Read the model definition and answer for the solid it produces. Units are mm, in the model's axes. A direction names the side the tool comes from. Coordinates: 2 decimals unless noted, no trailing zeros. Loops run counter-clockwise (first coordinate to the right, second up) from the corner with the lowest first, then second, coordinate; pieces in that order, holes last. Notation, with made-up numbers: (0, 4) -> (44, 4) arc R33 ccw to (44, 38) -> close; hole circle Ø4 at (27.25, -17.75). An arc over 180 degrees is marked (long way). Answer in a Markdown table with one row per item.
```python
from build123d import *

# Parameters (mm, degrees)
SKETCH28_W                                   = 80
SKETCH28_H                                   = 80
BOSS_EXTRUDE1_DEPTH                          = 10
CBORE_FOR_M10_CHEESE_HEAD_SCREW1_D           = 12
CBORE_FOR_M10_CHEESE_HEAD_SCREW1_CBORE_D     = 26
CBORE_FOR_M10_CHEESE_HEAD_SCREW1_CBORE_DEPTH = 5
SKETCH36_R                                   = 1
BOSS_EXTRUDE5_DEPTH                          = 10
SKETCH37_R                                   = 22.5
SKETCH37_R_2                                 = 15.5
CUT_EXTRUDE2_DEPTH                           = 6
CUT_EXTRUDE6_DEPTH                           = 6
SKETCH40_W                                   = 18.062589032
SKETCH40_H                                   = 3
BOSS_EXTRUDE7_DEPTH                          = 13
SKETCH41_R                                   = 33.75
SKETCH41_R_2                                 = 26.25
CUT_EXTRUDE7_DEPTH                           = 1.65
SKETCH42_W                                   = 9.8
SKETCH42_H                                   = 11.037342061
CUT_EXTRUDE8_DEPTH                           = 2
CUT_EXTRUDE11_DEPTH                          = 20
SKETCH45_W                                   = 2.851047628
SKETCH45_H                                   = 9.955339391
BOSS_EXTRUDE8_DEPTH                          = 14
BOSS_EXTRUDE9_START                          = -9.955339
BOSS_EXTRUDE9_DEPTH                          = 9.955339


with BuildPart() as part:
    # Sketch28 → Boss-Extrude1 (new body)
    with BuildSketch(Plane(origin=(0, 0, 0), x_dir=(1, 0, 0), z_dir=(0, 1, 0))):
        with Locations((1.944585414, 4.241283073)):
            Rectangle(SKETCH28_W, SKETCH28_H)
    extrude(amount=BOSS_EXTRUDE1_DEPTH)

    # CBORE for M10 Cheese Head Screw1 (through all)
    with Locations(Plane(origin=(0, 10, 0), x_dir=(1, 0, 0), z_dir=(0, 1, 0))):
        with Locations((1.944585414, 4.241283073)):
            CounterBoreHole(CBORE_FOR_M10_CHEESE_HEAD_SCREW1_D / 2, CBORE_FOR_M10_CHEESE_HEAD_SCREW1_CBORE_D / 2, CBORE_FOR_M10_CHEESE_HEAD_SCREW1_CBORE_DEPTH)

    # Sketch36 → Boss-Extrude5 (add)
    with BuildSketch(Plane.XZ):
        with Locations(Location((12.444585414, -16.741283073, 0), (0, 0, 270))):
            Circle(SKETCH36_R)
        with Locations(Location((12.444585414, -4.241283073, 0), (0, 0, 270))):
            Circle(SKETCH36_R)
        with Locations(Location((-8.555414586, -16.741283073, 0), (0, 0, 90))):
            Circle(SKETCH36_R)
        with Locations(Location((-8.555414586, -4.241283073, 0), (0, 0, 90))):
            Circle(SKETCH36_R)
    extrude(amount=BOSS_EXTRUDE5_DEPTH)

    # Sketch37 → Cut-Extrude2 (cut)
    with BuildSketch(Plane(origin=(0, 10, 0), x_dir=(1, 0, 0), z_dir=(0, 1, 0))):
        with Locations(Location((1.944585414, 4.241283073, 0), (0, 0, 270))):
            Circle(SKETCH37_R)
        with Locations(Location((1.944585414, 4.241283073, 0), (0, 0, 270))):
            Circle(SKETCH37_R_2, mode=Mode.SUBTRACT)
    extrude(amount=-CUT_EXTRUDE2_DEPTH, mode=Mode.SUBTRACT)

    # Sketch39 → Cut-Extrude6 (cut)
    with BuildSketch(Plane(origin=(0, 10, 0), x_dir=(1, 0, 0), z_dir=(0, 1, 0))):
        with BuildLine():
            Line((6.944585414, -35.758716927), (6.944585414, -17.696127895))
            ThreePointArc((6.944585414, -17.696127895), (1.944585414, -18.258716927), (-3.055414586, -17.696127895))
            Line((-3.055414586, -17.696127895), (-3.055414586, -35.758716927))
            Line((-3.055414586, -35.758716927), (1.944585414, -35.758716927))
            Line((1.944585414, -35.758716927), (6.944585414, -35.758716927))
        make_face()
    extrude(amount=-CUT_EXTRUDE6_DEPTH, mode=Mode.SUBTRACT)

    # Sketch40 → Boss-Extrude7 (add)
    with BuildSketch(Plane(origin=(-3.055414586, 0, 0), x_dir=(0, 0, -1), z_dir=(1, 0, 0))):
        with Locations((-26.727422411, 8.5)):
            Rectangle(SKETCH40_W, SKETCH40_H)
    extrude(amount=BOSS_EXTRUDE7_DEPTH)

    # Sketch41 → Cut-Extrude7 (cut)
    with BuildSketch(Plane(origin=(0, 10, 0), x_dir=(1, 0, 0), z_dir=(0, 1, 0))):
        with Locations(Location((1.944585414, 4.241283073, 0), (0, 0, 270))):
            Circle(SKETCH41_R)
        with Locations(Location((1.944585414, 4.241283073, 0), (0, 0, 270))):
            Circle(SKETCH41_R_2, mode=Mode.SUBTRACT)
    extrude(amount=-CUT_EXTRUDE7_DEPTH, mode=Mode.SUBTRACT)

    # Sketch42 → Cut-Extrude8 (cut)
    with BuildSketch(Plane.XZ):
        with Locations((1.966640169, -13.109663986)):
            Rectangle(SKETCH42_W, SKETCH42_H)
    extrude(amount=-CUT_EXTRUDE8_DEPTH, mode=Mode.SUBTRACT)

    # Sketch43 → Cut-Extrude11 (cut)
    with BuildSketch(Plane(origin=(0, 10, 0), x_dir=(1, 0, 0), z_dir=(0, 1, 0))):
        with BuildLine():
            ThreePointArc((-38.055414586, 4.241282966), (-26.339685871, 32.525554283), (1.944585414, 44.241283073))
            Line((1.944585414, 44.241283073), (-38.055414586, 44.241283073))
            Line((-38.055414586, 44.241283073), (-38.055414586, 4.241282966))
        make_face()
        with BuildLine():
            ThreePointArc((1.944585414, -35.758716927), (-26.339685795, -24.042988212), (-38.055414586, 4.241282966))
            Line((-38.055414586, 4.241282966), (-38.055414586, -35.758716927))
            Line((-38.055414586, -35.758716927), (1.944585414, -35.758716927))
        make_face()
        with BuildLine():
            Line((41.944585414, -35.758716927), (41.944585414, 4.241283073))
            ThreePointArc((41.944585414, 4.241283073), (30.228856662, -24.042988174), (1.944585414, -35.758716927))
            Line((1.944585414, -35.758716927), (41.944585414, -35.758716927))
        make_face()
        with BuildLine():
            Line((41.944585414, 44.241283073), (1.944585414, 44.241283073))
            ThreePointArc((1.944585414, 44.241283073), (30.228856662, 32.525554321), (41.944585414, 4.241283073))
            Line((41.944585414, 4.241283073), (41.944585414, 44.241283073))
        make_face()
    extrude(amount=-CUT_EXTRUDE11_DEPTH, mode=Mode.SUBTRACT)

    # Sketch45 → Boss-Extrude8 (add)
    with BuildSketch(Plane(origin=(0, 8.35, 0), x_dir=(1, 0, 0), z_dir=(0, 1, 0))):
        with Locations((-32.810971356, 5.43037333)):
            Rectangle(SKETCH45_W, SKETCH45_H)
    extrude(amount=BOSS_EXTRUDE8_DEPTH)

    # Sketch46 → Boss-Extrude9 (add)
    with BuildSketch(Plane.XY.offset(-0.452703634).offset(BOSS_EXTRUDE9_START)):
        Polygon((-31.385447542, 22.35), (-31.385447542, 20.057188555), (-29.944471524, 20.057188555), align=None)
    extrude(amount=BOSS_EXTRUDE9_DEPTH)


solid = part.part
```
1. A cutting plane is placed at C-C on y = -5. Give the vertices of the cut face in (x, z), and give its area (3 significant figures).
A:
| item | result |
|---|---|
| outline | circle Ø2 at (-8.56, -16.74); circle Ø2 at (-8.56, -4.24); circle Ø2 at (12.44, -16.74); circle Ø2 at (12.44, -4.24) |
| area | 12.6 mm2 |
2. A cutting plane is placed at B-B on z = 10. Give the vertices of the cut face in (x, y), and give its area (3 significant figures).
A:
| item | result |
|---|---|
| outline | (-35.43, 0) -> (39.32, 0) -> (39.32, 10) -> (32.54, 10) -> (32.54, 8.35) -> (24, 8.35) -> (24, 10) -> (19.36, 10) -> (19.36, 4) -> (8.06, 4) -> (8.06, 10) -> (-4.17, 10) -> (-4.17, 4) -> (-15.47, 4) -> (-15.47, 10) -> (-20.11, 10) -> (-20.11, 8.35) -> (-28.65, 8.35) -> (-28.65, 10) -> (-35.43, 10) -> close |
| area | 584 mm2 |
3. A cutting plane is placed at D-D on y = 15. Give the vertices of the cut face in (x, z).
A:
| item | result |
|---|---|
| outline | (-34.24, -10.41) -> (-31.39, -10.41) -> (-31.39, -0.45) -> (-34.24, -0.45) -> close |
4. The mould has two halves that part along Y. Classify faces 1 (the cylindrical face through (9.829, 9.187, 20.797)), 2 (the flat face through (2, 7, 27)), 3 (the flat face through (15, 10, -1)): pulls with the +Y half, pulls with the -Y half, needs draft (parallel to the pull), parting line crosses it, or undercut.
A:
| item | result |
|---|---|
| face 1 | needs draft |
| face 2 | undercut |
| face 3 | pulls with the +Y half |
5. Given pin 1 Ø12 at (y, z) = (3, -31) entering from +X; pin 2 Ø1.3 at (x, y) = (-33, 14) entering from +Z; pin 3 Ø13 at (x, z) = (2, -5.5) entering from +Y, each flat-ended and moving along its own axis, determine where each tip first touches the part or whether it passes through.
A:
| item | result |
|---|---|
| pin 1 | stops at x = 36.14 |
| pin 2 | stops at z = -0.45 |
| pin 3 | stops at y = 5 |
6. A cutting plane is placed at A-A on x = -29. Give the vertices of the cut face in (y, z), and give its area (3 significant figures).
A:
| item | result |
|---|---|
| outline | (0, -29.59) -> (10, -29.59) -> (10, -17.71) -> (8.35, -17.71) -> (8.35, 9.23) -> (10, 9.23) -> (10, 21.1) -> (0, 21.1) -> close |
| area | 462 mm2 |
7. A tool of negligible diameter and unlimited length cuts with its end or side. For faces 4 (the flat face through (-2.933, 1, -13)), 5 (the cylindrical face through (-0.87, 7.54, 8.45)), 6 (the flat face through (7, 4, 11)), from which of +Z, -Z, +X, -X, +Y, -Y can it reach the whole face along a straight path? Write none if from no direction.
A:
| item | result |
|---|---|
| face 4 | -Y |
| face 5 | +Y |
| face 6 | none |
8. Find the intervals of material crossed by probe 1 along Z at (x, y) = (-0.5, 8.5); probe 2 along Y at (x, z) = (31.5, -0.5); probe 3 along Y at (x, z) = (-8, -7), in increasing order.
A:
| item | result |
|---|---|
| probe 1 | z = -44.17 to -37.9, -30.38 to -26.61, -19.55 to -17.01, 8.53 to 11.06, 17.7 to 21.89, 29.42 to 35.68 |
| probe 2 | y = 0 to 8.35 |
| probe 3 | y = 0 to 5 |
